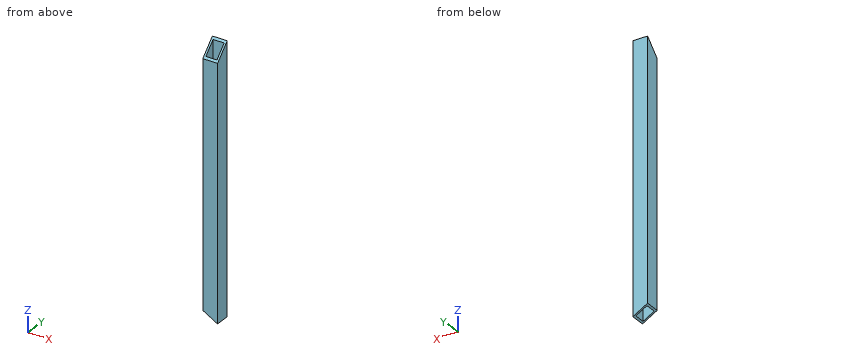
Autodesk Inventor part; units mm, degrees
ref_plane "YZ Plane" through (0, 0, 0) normal (1, 0, 0) x (0, 1, 0)
ref_plane "XZ Plane" through (0, 0, 0) normal (0, 1, 0) x (-1, 0, 0)
ref_plane "XY Plane" through (0, 0, 0) normal (0, 0, 1) x (1, 0, 0)
sketch "Sketch1" plane through (0, 0, 0) normal (0, 0, 1) x (1, 0, 0)
  line L0 (-17.78, 0) -> (17.78, 0)
  line L1 (0, -17.78) -> (0, 17.78)
  line L2 (-12.7, 12.7) -> (12.7, 12.7)
  line L3 (12.7, 12.7) -> (12.7, -12.7)
  line L4 (12.7, -12.7) -> (-12.7, -12.7)
  line L5 (-12.7, -12.7) -> (-12.7, 12.7)
  line L6 (9.525, 9.525) -> (-9.525, 9.525)
  line L7 (-9.525, 9.525) -> (-9.525, -9.525)
  line L8 (-9.525, -9.525) -> (9.525, -9.525)
  line L9 (9.525, -9.525) -> (9.525, 9.525)
  point P0 (0, 0)
  point P1 (-12.7, 0)
  point P2 (0, 12.7)
  dimension "d0" = 25.4
  dimension "d1" = 3.175
extrude "Base" add sketch "Sketch1" along normal mid plane 457.2 contours L5 L2 L1 L6 L7 L0 | L0 L7 L8 L1 L4 L5 | L1 L8 L9 L0 L3 L4 | L2 L3 L0 L9 L6 L1
sketch "Sketch5" plane through (-12.7, -12.7, 228.6) normal (-1, 0, 0) x (0, 0, 1)
  line L0 (0, 0) -> (0, 25.4)
  line L1 (-457.2, 25.4) -> (0, 25.4)
  line L2 (0, 0) -> (-457.2, 0)
  line L3 (0, 25.4) -> (-25.4, 0)
  line L4 (-228.6, 25.4) -> (-228.6, 0) construction
  point P0 (-228.6, 12.7)
  dimension "d13" = 45
extrude "Extrusion5" cut sketch "Sketch5" against normal through all
sketch "Sketch6" plane through (-12.7, 12.7, -228.6) normal (0, 1, 0) x (1, 0, 0)
  line L0 (25.4, 0) -> (0, 0)
  line L1 (0, 0) -> (0, -457.2)
  line L2 (25.4, 0) -> (0, -14.6647)
  point P0 (12.7, -228.6)
  dimension "d16" = 30
extrude "Extrusion6" cut sketch "Sketch6" against normal through all
properties part number "tubing_template_0.125" material "Aluminum-6061"
The model under review builds one solid part; all positions refer to its coordinate system, in mm. Round coordinates to 2 decimals unless told otherwise and drop trailing zeros. Write each loop counter-clockwise with the first axis right and the second up, starting at its lowest first coordinate (ties: lowest second). Pieces come first, ordered by that corner, then holes. Notation, with made-up numbers: M 34,6 L 70,6 A19 ccw 70,43 Z; hole C 40.25,-6 d6. An arc over 180 degrees is marked long. Answer as CSV lines item,"result". Start each with the question number.
Q1. Wall thickness on line 1 along X through (y, z) = (6.5, -207.5) (3 decimals); line 2 along Z through (x, y) = (-9.75, 4): over which ranges is each line inside the solid? List them lowest first.
Q2. Consider section B-B, the plane z = -153. Give the boundary of the cut face in (x, y) (3 decimals), then the cut area to 3 significant figures.
Q3. Consider section A-A, the plane y = -1.25. Give the boundary of the cut face in (x, z) (3 decimals), then the cut area to 3 significant figures.
Q4. Consider section C-C, the plane x = -0.75. Give the boundary of the cut face in (y, z) (3 decimals), then the cut area to 3 significant figures.
Result set:
1,line 1,"x = -12.7 to -9.525, 9.525 to 12.7"
1,line 2,"z = -215.64 to 219.9"
2,outline,"M -12.7,-12.7 L 12.7,-12.7 L 12.7,12.7 L -12.7,12.7 Z; hole M -9.525,-9.525 L 9.525,-9.525 L 9.525,9.525 L -9.525,9.525 Z"
2,area,"282 mm²"
3,outline,"M -12.7,-213.935 L -9.525,-215.768 L -9.525,214.65 L -12.7,214.65 Z; M 9.525,-226.767 L 12.7,-228.6 L 12.7,214.65 L 9.525,214.65 Z"
3,area,"2,770 mm²"
4,outline,"M -12.7,-220.835 L -9.525,-220.835 L -9.525,206.375 L -12.7,203.2 Z; M 9.525,-220.835 L 12.7,-220.835 L 12.7,228.6 L 9.525,225.425 Z"
4,area,"2,770 mm²"
